Autodesk Inventor part; units mm, degrees
ref_plane "YZ Plane" through (0, 0, 0) normal (1, 0, 0) x (0, 1, 0)
ref_plane "XZ Plane" through (0, 0, 0) normal (0, 1, 0) x (-1, 0, 0)
ref_plane "XY Plane" through (0, 0, 0) normal (0, 0, 1) x (1, 0, 0)
sketch "Sketch1" plane through (0, 0, 0) normal (0, 0, 1) x (1, 0, 0)
  line L0 (-776, -450) -> (776, -450)
  line L1 (776, -450) -> (776, 0)
  line L2 (776, 0) -> (-776, 0)
  line L3 (-776, 0) -> (-776, -450)
  point P0 (0, 0)
  point P1 (0, 0)
  dimension "d0" = 450
  dimension "d1" = 1552
extrude "Plate1" add sketch "Sketch1" along normal blind 2
sketch "Sketch2" plane through (0, 0, 2) normal (0, 0, 1) x (1, 0, 0)
  line L0 (776, -450) -> (-776, -450)
  line L1 (776, 0) -> (776, -450)
  line L2 (-776, 0) -> (776, 0)
  line L3 (-776, -450) -> (-776, 0)
  line L4 (775.9, 0) -> (762.994, -167.1926)
  line L5 (762.994, -167.1926) -> (538, -450)
  line L6 (776, -450) -> (-776, -450)
  point P0 (0, 0)
  point P1 (0, -450)
  dimension "d3" = 0.1
  dimension "d9" = 167.1926
  dimension "d13" = 85.586
  dimension "d14" = 51.495
  dimension "d15" = 538
extrude "Extrusion1" cut sketch "Sketch2" against normal through all contours L0 L5 L4 L2 L1
mirror "Mirror1" about plane through (0, 0, 0) normal (1, 0, 0) of "Extrusion1"
equation "\"d2\" = Thickness"
equation "\"BendReliefWidth\" = Thickness"
equation "\"BendReliefDepth\" = 0.5 * Thickness"
equation "\"CornerReliefSize\" = 4 * Thickness"
equation "\"MinimumRemnant\" = 2 * Thickness"
equation "\"TransitionRadius\" = BendRadius"
equation "\"JacobiRadiusSize\" = BendRadius"
equation "\"GapSize\" = Thickness"
properties part number "MSC 704 FACE 4" material "Stainless Steel"
Model file for the job. Use its own axes, mm. Round coordinates to 2 decimals unless told otherwise and drop trailing zeros. Loops run counter-clockwise (first coordinate to the right, second up) from the corner with the lowest first, then second, coordinate; pieces in that order, holes last.
1. Band-saw the part on B-B, the plane x = 600. List the corners of the cut face in (y, z).
Check values:
outline: (-372.07, 0) - (0, 0) - (0, 2) - (-372.07, 2) - close
2. Drop a flat-ended pin along its axis: P1, Ø1, axis at x = 602, z = 1, coming from the -Y side. Give the stop position or say it passes through.
Check values:
P1: stops at y = -370.18
3. Band-saw the part on C-C, the plane y = -325. List the corners of the cut face in (x, z), and give its area (3 significant figures).
Check values:
outline: (-637.45, 0) - (637.45, 0) - (637.45, 2) - (-637.45, 2) - close
area: 2,550 mm2
4. Band-saw the part on A-A, the plane z = 1.5. List the corners of the cut face in (x, y).
Check values:
outline: (-775.9, 0) - (-762.99, -167.19) - (-538, -450) - (538, -450) - (762.99, -167.19) - (775.9, 0) - close
5. Wall check: probe 1 along X at (y, z) = (-423, 1.4); probe 2 along X at (y, z) = (-322, 1); probe 3 along Y at (x, z) = (-625, 1.45). Give the ranges that are in metal, low to high.
Check values:
probe 1: x = -559.48 to 559.48
probe 2: x = -639.83 to 639.83
probe 3: y = -340.64 to 0
